Can you work these out from the model? Positions are in its coordinate system, mm. A direction names the side the tool comes from. Give positions to 0.01 mm unless a question says otherwise; leave off trailing zeros. Write each loop counter-clockwise with the first axis right and the second up, starting at its lowest first coordinate (ties: lowest second). Pieces come first, ordered by that corner, then holes.
Autodesk Inventor part; units mm, degrees
ref_plane "YZ Plane" through (0, 0, 0) normal (1, 0, 0) x (0, 1, 0)
ref_plane "XZ Plane" through (0, 0, 0) normal (0, 1, 0) x (-1, 0, 0)
ref_plane "XY Plane" through (0, 0, 0) normal (0, 0, 1) x (1, 0, 0)
sketch "Sketch1" plane through (0, 0, 0) normal (0, 0, 1) x (1, 0, 0)
  circle A0 centre (0, 0) radius 3.175
  dimension "d0" = 6.35
extrude "Extrusion1" add sketch "Sketch1" along normal blind 12.7
sketch "Sketch2" plane through (0, 0, 12.7) normal (0, 0, 1) x (1, 0, 0)
  circle A0 centre (0, 0) radius 3.175
  line L0 (0, 6.2325) -> (5.3975, 3.1162)
  line L1 (5.3975, 3.1162) -> (5.3975, -3.1162)
  line L2 (5.3975, -3.1162) -> (0, -6.2325)
  line L3 (0, -6.2325) -> (-5.3975, -3.1162)
  line L4 (-5.3975, -3.1162) -> (-5.3975, 3.1162)
  line L5 (-5.3975, 3.1162) -> (0, 6.2325)
  dimension "d3" = 10.795
extrude "Extrusion2" add sketch "Sketch2" along normal blind 3.81 contours A0 | L0 L1 L2 L3 L4 L5
thread "Thread1"
properties part number "Bolt .5 1764"
1) For faces 1 (the face through (2, -3, 12.7)), 2 (the face through (-2.661, -4.696, 14.578)), which set-ups out of +Z, -Z, +X, -X, +Y, -Y let a thin tool reach every point of the face, with its end or its side?
Values follow:
face 1: -Z
face 2: +Z, -Z, -X, -Y
2) Suppose I cut it at A-A on y = 0. Write out the boundary of the cut face in (x, z) (1 decimal), plus the area to 3 significant figures.
Values follow:
outline: (-5.4, 12.7) - (-3.2, 12.7) - (-3.2, 0) - (3.2, 0) - (3.2, 12.7) - (5.4, 12.7) - (5.4, 16.5) - (-5.4, 16.5) - close
area: 122 mm2
3) Please list where these lines run through material, in increasing order: L1, parallel to Z at x = -0.25, y = 4.75; L2, parallel to X at y = 1.5, z = 12; L3, parallel to X at y = 2.75, z = 9.
Values follow:
L1: z = 12.7 to 16.51
L2: x = -2.8 to 2.8
L3: x = -1.59 to 1.59
4) Suppose I cut it at C-C on z = 1.5. Write out the boundary of the cut face in (x, y) (3 decimals).
Values follow:
outline: circle Ø6.35 at (0, 0)
5) For pin 1 Ø1.5 at (x, y) = (-4, -5) entering from +Z; pin 2 Ø1.5 at (x, z) = (2.5, 14) entering from -Y, each with a flat end and sliding along its axis, tell me the tip position at first contact or that it passes through.
Values follow:
pin 1: passes through
pin 2: stops at y = -5.22
6) Suppose I cut it at B-B on x = -0.5. Write out the boundary of the cut face in (y, z).
Values follow:
outline: (-5.94, 12.7) - (-3.14, 12.7) - (-3.14, 0) - (3.14, 0) - (3.14, 12.7) - (5.94, 12.7) - (5.94, 16.51) - (-5.94, 16.51) - close
